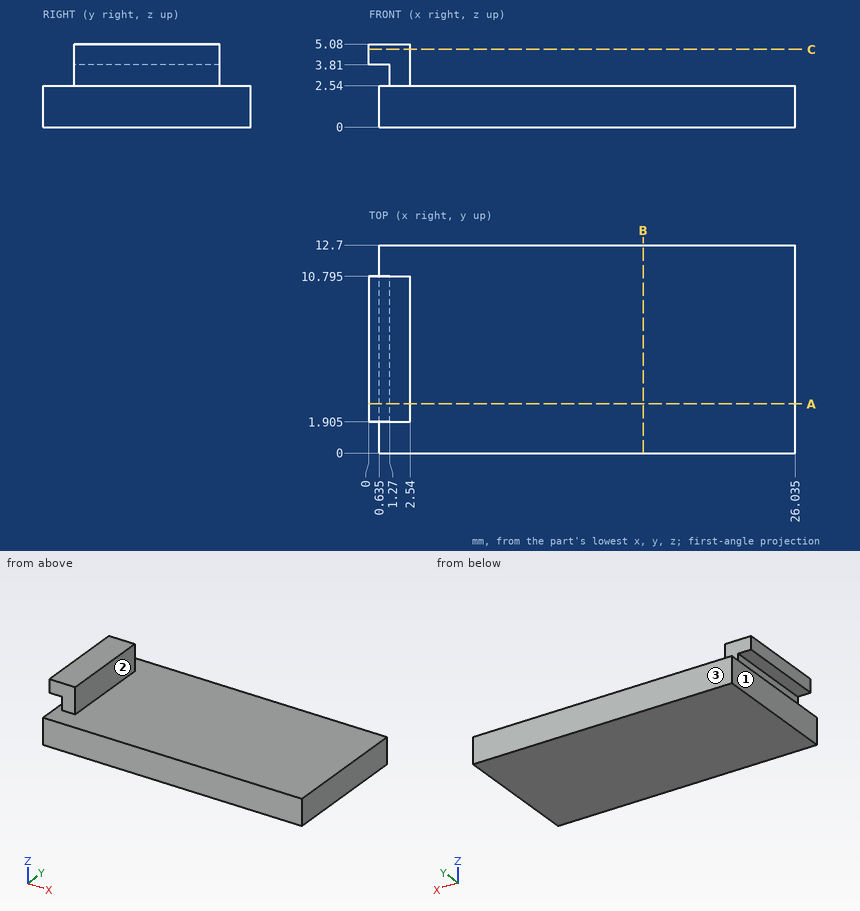
Verification items for this drawing (mm, ordinates from the low corner). A direction names the side the tool comes from. Round coordinates to 2 decimals unless told otherwise and drop trailing zeros. Order: outer loops, then holes, each group sorted by start corner. A loop starts at its lowest first (then second) coordinate and runs counter-clockwise, first axis right, second up. Notation, with made-up numbers: (-14, -28) - (36, -28) arc R14 cw to (36, -4) - close; hole circle Ø1 at (29.25, -3). An arc over 180 degrees is marked (long way). Answer as CSV lines item,"result". Start each with the question number.
1) Tool access check on the marked faces 1, 2 and 3. Record the directions out of +Z, -Z, +X, -X, +Y, -Y that give a thin tool (end or side, any length) a straight path to the whole face; none if there is none.
2) Depth check by flat-ended pin: pin 1 (3 mm diameter, centred on y = 4, z = 0.5, fed in from -X) (3 decimals); pin 2 (2 mm diameter, centred on x = 1, z = 3.5, fed in from -Y); pin 3 (1.5 mm diameter, centred on x = 12.5, y = 9, fed in from +Z); pin 4 (0.6 mm diameter, centred on y = 7.5, z = 3, fed in from -X). Enter the tip coordinate at first touch or a pass-through.
3) Section check A-A (y = 3). Record the cut outline in (x, z) (3 decimals).
4) Scan lines: probe 1 along Z at (x, y) = (8.75, 2); probe 2 along X at (y, z) = (12, 1.75) (3 decimals). Record each from-to range of solid material in increasing order.
5) Section check B-B (x = 16.75). Record the cut outline in (y, z).
6) Section check C-C (z = 4.75). Record the cut outline in (x, y) (3 decimals), then the cut area to 3 significant figures.
Determined:
1,face 1,"-Z, -X, +Y, -Y"
1,face 2,"+Z, +X, +Y, -Y"
1,face 3,"+Z, -Z, +X, -X, +Y"
2,pin 1,"x = 0.635"
2,pin 2,"y = 0"
2,pin 3,"z = 2.54"
2,pin 4,"x = 1.27"
3,outline,"(0, 3.81) - (1.27, 3.81) - (1.27, 2.54) - (0.635, 2.54) - (0.635, 0) - (26.035, 0) - (26.035, 2.54) - (2.54, 2.54) - (2.54, 5.08) - (0, 5.08) - close"
4,probe 1,"0 to 2.54"
4,probe 2,"0.635 to 26.035"
5,outline,"(0, 0) - (12.7, 0) - (12.7, 2.54) - (0, 2.54) - close"
6,outline,"(0, 1.905) - (2.54, 1.905) - (2.54, 10.795) - (0, 10.795) - close"
6,area,"22.6 mm^2"
